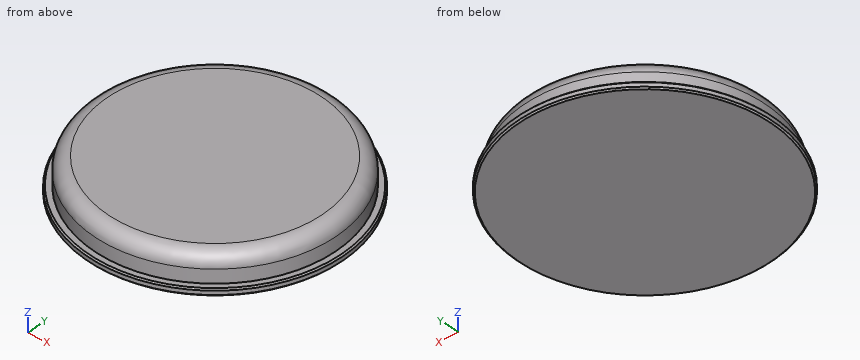
from build123d import *

# Parameters (mm, degrees)
SKETCH_R     = 94
PAD_DEPTH    = 5
SKETCH001_R  = 89
PAD001_DEPTH = 20
FILLET_R     = 10
CHAMFER_SIZE = 1


with BuildPart() as part:
    # Sketch → Pad (new body)
    with BuildSketch(Plane.XY):
        Circle(SKETCH_R)
    extrude(amount=PAD_DEPTH)

    # Sketch001 → Pad001 (new body)
    with BuildSketch(Plane.XY.offset(5)):
        Circle(SKETCH001_R)
    extrude(amount=PAD001_DEPTH)

    # Fillet
    fillet_edges = [part.edges().sort_by_distance(p)[0] for p in [
        (-89, 0, 25),
    ]]
    fillet(fillet_edges, radius=FILLET_R)

    # Chamfer
    chamfer_edges = [part.edges().sort_by_distance(p)[0] for p in [
        (-94, 0, 0),
        (-94, 0, 5),
    ]]
    chamfer(chamfer_edges, length=CHAMFER_SIZE)


solid = part.part
CAD build for the part. Positions are in the model's coordinates, mm. Round coordinates to 2 decimals unless told otherwise and drop trailing zeros. Write each loop counter-clockwise with the first axis right and the second up, starting at its lowest first coordinate (ties: lowest second). Pieces come first, ordered by that corner, then holes.
(1) Probe line 1 along Z through (x, y) = (22, 86.5); line 2 along Y through (x, z) = (39, 16.25); line 3 along Y through (x, z) = (80, 21.25). List the from-to ranges inside material, lowest first.
(2) Slice it at C-C, the plane z = 10.5. Write the cut outline in (x, y).
(3) Drop flat-ended pins along their axis: P1, Ø8, axis at y = -61.5, z = 6, coming from the -X side; P2, Ø10, axis at y = 12.5, z = 17, coming from the +X side; P3, Ø4, axis at y = -41.5, z = 9, coming from the +X side. Give the stop position or say it passes through.
(4) Slice it at A-A, the plane x = 0. Write the cut outline in (y, z), and give its area (3 significant figures).
(5) Slice it at D-D, the plane z = 21.75. Write the cut outline in (x, y).
From the geometry:
1. line 1: z = 0 to 5
1. line 2: y = -79.91 to 79.91
1. line 3: y = -33.69 to 33.69
2. outline: circle Ø178 at (0, 0)
3. P1: stops at x = -73.94
3. P2: stops at x = 88.65
3. P3: stops at x = 79.75
4. outline: (-94, 1) - (-93, 0) - (93, 0) - (94, 1) - (94, 4) - (93, 5) - (89, 5) - (89, 15) arc R10 ccw to (79, 25) - (-79, 25) arc R10 ccw to (-89, 15) - (-89, 5) - (-93, 5) - (-94, 4) - close
4. area: 4,460 mm2
5. outline: circle Ø172.76 at (0, 0)
